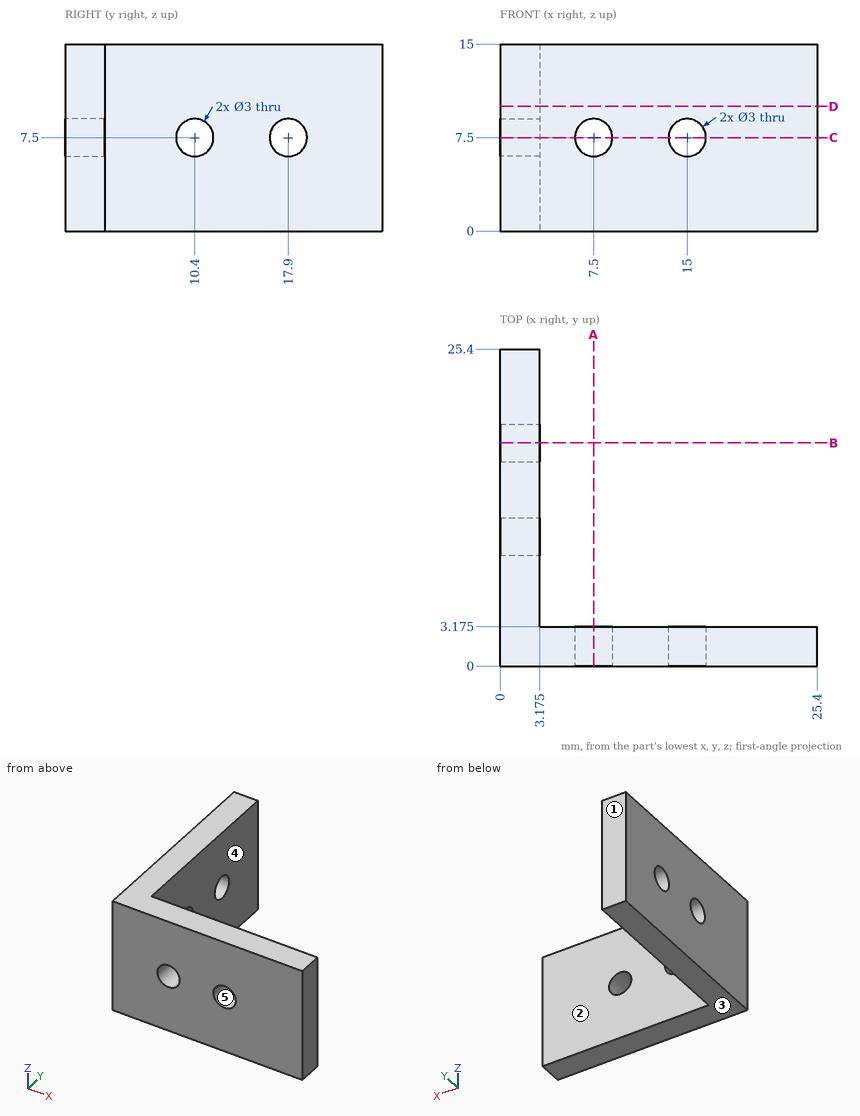
Can you work these out from the drawing? Everything is in mm from the part's minimum corner. A direction names the side the tool comes from. Coordinates: 2 decimals unless noted, no trailing zeros. Loops run counter-clockwise (first coordinate to the right, second up) from the corner with the lowest first, then second, coordinate; pieces in that order, holes last.
1. Imagine slicing it at C-C, the plane z = 7.5. Please give me the cut outline in (x, y) (3 decimals).
2. Imagine slicing it at A-A, the plane x = 7.5. Please give me the cut outline in (y, z) (3 decimals).
3. I need wall thicknesses on L1, parallel to Y at x = 2.5, z = 7.5; L2, parallel to X at y = 0.7, z = 7.5; L3, parallel to X at y = 7, z = 7.5 (3 decimals). Which ranges of each line are inside material? Lowest first, please.
4. If we mould it in two halves opening along X, with no side actions, what happens to the marked faces 3, 4 and 5? For each: pulls with the +X half, pulls with the -X half, needs draft (parallel to the pull), parting line crosses it, or undercut.
5. For P1, Ø3, axis at y = 9.5, z = 7.5, coming from the +X side (3 decimals); P2, Ø4, axis at x = 15, z = 7.5, coming from the +Y side (3 decimals), each with a flat end and sliding along its axis, tell me the tip position at first contact or that it passes through.
6. Imagine slicing it at D-D, the plane z = 10. Please give me the cut outline in (x, y) (3 decimals), and give its area (3 significant figures).
7. For the marked faces 1 and 2, which set-ups out of +Z, -Z, +X, -X, +Y, -Y let a thin tool reach every point of the face, with its end or its side?
Taken from the geometry:
1. outline: (0, 0) - (6, 0) - (6, 3.175) - (3.175, 3.175) - (3.175, 8.9) - (0, 8.9) - close; (0, 11.9) - (3.175, 11.9) - (3.175, 16.4) - (0, 16.4) - close; (0, 19.4) - (3.175, 19.4) - (3.175, 25.4) - (0, 25.4) - close; (9, 0) - (13.5, 0) - (13.5, 3.175) - (9, 3.175) - close; (16.5, 0) - (25.4, 0) - (25.4, 3.175) - (16.5, 3.175) - close
2. outline: (0, 0) - (3.175, 0) - (3.175, 6) - (0, 6) - close; (0, 9) - (3.175, 9) - (3.175, 15) - (0, 15) - close
3. L1: y = 0 to 8.9, 11.9 to 16.4, 19.4 to 25.4
3. L2: x = 0 to 6, 9 to 13.5, 16.5 to 25.4
3. L3: x = 0 to 3.175
4. face 3: needs draft
4. face 4: pulls with the +X half
4. face 5: undercut
5. P1: stops at x = 3.175
5. P2: stops at y = 3.175
6. outline: (0, 0) - (25.4, 0) - (25.4, 3.175) - (3.175, 3.175) - (3.175, 25.4) - (0, 25.4) - close
6. area: 151 mm2
7. face 1: +Z, -Z, +X, -X, +Y
7. face 2: +Z, -Z, +X, +Y
